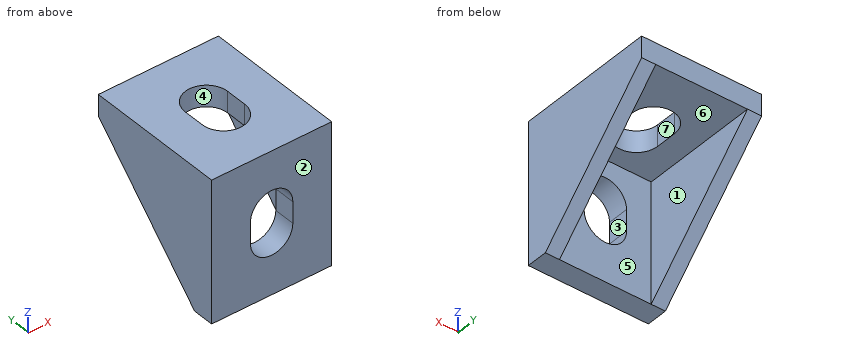
Autodesk Inventor part; units mm, degrees
ref_plane "YZ Plane" through (0, 0, 0) normal (1, 0, 0) x (0, 1, 0)
ref_plane "XZ Plane" through (0, 0, 0) normal (0, 1, 0) x (-1, 0, 0)
ref_plane "XY Plane" through (0, 0, 0) normal (0, 0, 1) x (1, 0, 0)
sketch "Sketch1" plane through (0, 0, 0) normal (0, 1, 0) x (-1, 0, 0)
  line L0 (0, 0) -> (-17, 0)
  line L1 (-17, 0) -> (-17, -20)
  line L2 (-17, -20) -> (0, -20)
  line L3 (0, -20) -> (0, 0)
  dimension "d0" = 17
  dimension "d1" = 20
extrude "Extrusion1" add sketch "Sketch1" along normal blind 3
sketch "Sketch2" plane through (0, 3, 0) normal (0, 1, 0) x (1, 0, 0)
  line L0 (17, 0) -> (17, 20)
  line L1 (17, 20) -> (0, 20)
  line L2 (0, 20) -> (0, 0)
  line L3 (0, 0) -> (17, 0)
  line L4 (8.5, 14.5) -> (8.5, 14.5)
  line L5 (5.5, 11.5) -> (5.5, 8.5)
  line L6 (8.5, 5.5) -> (8.5, 5.5)
  line L7 (11.5, 8.5) -> (11.5, 11.5)
  arc A0 (8.5, 14.5) -> (5.5, 11.5) centre (8.5, 11.5) ccw
  arc A1 (11.5, 11.5) -> (8.5, 14.5) centre (8.5, 11.5) ccw
  arc A2 (5.5, 8.5) -> (8.5, 5.5) centre (8.5, 8.5) ccw
  arc A3 (8.5, 5.5) -> (11.5, 8.5) centre (8.5, 8.5) ccw
  point P0 (5.5, 5.5)
  point P1 (5.5, 14.5)
  point P2 (11.5, 5.5)
  dimension "d6" = 6
  dimension "d7" = 9
  dimension "d8" = 3
extrude "Extrusion2" cut sketch "Sketch2" against normal blind 3 contours A0 A1 L7 A3 A2 L5
sketch "Sketch3" plane through (0, 3, 0) normal (0, 1, 0) x (1, 0, 0)
  line L0 (11.5, 11.5) -> (11.5, 8.5)
  arc A0 (5.5, 8.5) -> (11.5, 8.5) centre (8.5, 8.5) ccw
  line L1 (5.5, 8.5) -> (5.5, 11.5)
  arc A1 (11.5, 11.5) -> (5.5, 11.5) centre (8.5, 11.5) ccw
  line L2 (17, 0) -> (17, 20)
  line L3 (17, 20) -> (0, 20)
  line L4 (0, 20) -> (0, 0)
  line L5 (0, 0) -> (17, 0)
  line L6 (0, 20) -> (0, 0)
  line L7 (0, 0) -> (17, 0)
  line L8 (17, 0) -> (17, 3)
  line L9 (17, 3) -> (0, 3)
  line L10 (0, 3) -> (0, 0)
  dimension "d11" = 3
extrude "Extrusion3" add sketch "Sketch3" along normal blind 17 contours L5 L4 L9 L2
sketch "Sketch4" plane through (0, 0, 0) normal (0, 0, 1) x (1, 0, 0)
  line L0 (0, 0) -> (17, 0)
  line L1 (17, 0) -> (17, 20)
  line L2 (0, 20) -> (17, 20)
  line L3 (0, 0) -> (0, 20)
  line L4 (8.5, 5.5) -> (8.5, 5.5)
  line L5 (11.5, 8.5) -> (11.5, 11.5)
  line L6 (8.5, 14.5) -> (8.5, 14.5)
  line L7 (5.5, 11.5) -> (5.5, 8.5)
  line L8 (5.5, 5.5) -> (11.5, 14.5) construction
  line L9 (11.5, 5.5) -> (5.5, 14.5) construction
  arc A0 (8.5, 14.5) -> (5.5, 11.5) centre (8.5, 11.5) ccw
  arc A1 (11.5, 11.5) -> (8.5, 14.5) centre (8.5, 11.5) ccw
  arc A2 (5.5, 8.5) -> (8.5, 5.5) centre (8.5, 8.5) ccw
  arc A3 (8.5, 5.5) -> (11.5, 8.5) centre (8.5, 8.5) ccw
  point P0 (8.5, 10)
  dimension "d14" = 6
  dimension "d15" = 9
  dimension "d16" = 3
extrude "Extrusion4" cut sketch "Sketch4" against normal blind 3 contours A3 A2 L7 A0 A1 L5
sketch "Sketch5" plane through (17, 0, 0) normal (1, 0, 0) x (0, 0, -1)
  line L0 (0, 0) -> (20, 0)
  line L1 (20, 0) -> (20, 3)
  line L2 (3, 3) -> (20, 3)
  line L3 (3, 3) -> (3, 20)
  line L4 (0, 20) -> (3, 20)
  line L5 (0, 0) -> (0, 20)
  line L6 (20, 3) -> (3, 20)
extrude "Extrusion5" add sketch "Sketch5" against normal blind 2 contours L2 L3 L6
sketch "Sketch6" plane through (0, 0, -20) normal (-1, 0, 0) x (0, 0, 1)
  line L0 (17, 3) -> (0, 3)
  line L1 (17, 3) -> (17, 20)
  line L2 (0, 3) -> (17, 20)
  line L3 (0, 0) -> (20, 0)
  line L4 (20, 0) -> (20, 20)
  line L5 (17, 20) -> (20, 20)
  line L6 (17, 3) -> (17, 20)
  line L7 (0, 3) -> (17, 3)
  line L8 (0, 0) -> (0, 3)
extrude "Extrusion6" add sketch "Sketch6" against normal blind 2 contours L0 L2 L1
properties part number "ANGULOESQUINA"
For this review, take the finished solid that the model builds, in its own axes (mm). Face numbers are marked on the shaded views. A direction names the side the tool comes from. Round coordinates to 2 decimals unless told otherwise and drop trailing zeros. Write each loop counter-clockwise with the first axis right and the second up, starting at its lowest first coordinate (ties: lowest second). Pieces come first, ordered by that corner, then holes. Notation, with made-up numbers: (38.5, 0.5) - (85.5, 0.5) arc R26 cw to (85.5, 34.5) - close; hole circle Ø8 at (23.5, 22). An arc over 180 degrees is marked (long way). Put each result on its own line as item: value.
Q1. Wall thickness on probe 1 along X at (y, z) = (10.75, -4); probe 2 along X at (y, z) = (9.75, -0.75); probe 3 along Z at (x, y) = (6, 14.25): over which ranges is each line inside the solid? List them lowest first.
Solved:
probe 1: x = 0 to 2, 15 to 17
probe 2: x = 0 to 5.5, 11.5 to 17
probe 3: z = -3 to 0
Q2. Machinability: for the marked faces 1, 2, 3 and 4, which of the approach directions +Z, -Z, +X, -X, +Y, -Y give a long, thin tool a straight path to every point of the face, cutting with its end or side? Answer none if there is none.
Solved:
face 1: -Z, +Y
face 2: +Z, -Z, +X, -X, -Y
face 3: +Y, -Y
face 4: +Z, -Z
Q3. Insertion check: pin 1 Ø1.5 at (x, z) = (12, -12.5) entering from +Y. The pin has a flat end and moves straight along its axis. Give the tip position at first contact, or say it passes through.
Solved:
pin 1: stops at y = 3
Q4. We need section A-A (y = 6.5). Give the boundary of the cut face in (x, z), and give its area (3 significant figures).
Solved:
outline: (0, -16.5) - (2, -16.5) - (2, -3) - (6.26, -3) - (6.26, 0) - (0, 0) - close; (10.74, -3) - (15, -3) - (15, -16.5) - (17, -16.5) - (17, 0) - (10.74, 0) - close
area: 91.6 mm2
Q5. We need section C-C (z = -4.25). Give the boundary of the cut face in (x, y), and give its area (3 significant figures).
Solved:
outline: (0, 0) - (17, 0) - (17, 18.75) - (15, 18.75) - (15, 3) - (2, 3) - (2, 18.75) - (0, 18.75) - close
area: 114 mm2
Q6. We need section B-B (x = 8.5). Give the boundary of the cut face in (y, z).
Solved:
outline: (0, -20) - (3, -20) - (3, -14.5) - (0, -14.5) - close; (0, -5.5) - (3, -5.5) - (3, -3) - (5.5, -3) - (5.5, 0) - (0, 0) - close; (14.5, -3) - (20, -3) - (20, 0) - (14.5, 0) - close
Q7. Mouldability with a two-part tool opening along Y and no side actions: class the marked faces 5, 6 and 7 as released by +Y, released by -Y, zero draft, split by the parting line, or undercut.
Solved:
face 5: released by +Y
face 6: zero draft
face 7: undercut
Q8. We need section D-D (z = -14). Give the boundary of the cut face in (x, y), and give its area (4 significant figures).
Solved:
outline: (0, 0) - (6.84, 0) - (6.84, 3) - (2, 3) - (2, 9) - (0, 9) - close; (10.16, 0) - (17, 0) - (17, 9) - (15, 9) - (15, 3) - (10.16, 3) - close
area: 65.05 mm2
